Autodesk Inventor part; units mm, degrees
ref_plane "Work Plane1" through (6.76, 0, 0) normal (1, 0, 0) x (0, 1, 0)
ref_plane "XZ Plane" through (0, 0, 0) normal (0, 1, 0) x (-1, 0, 0)
ref_plane "XY Plane" through (0, 0, 0) normal (0, 0, 1) x (1, 0, 0)
sketch "Sketch1" plane through (0, 0, 0) normal (0, 1, 0) x (-1, 0, 0)
  circle A0 centre (0, 0) radius 11.5
  dimension "d0" = 23
extrude "Extrusion1" add sketch "Sketch1" along normal blind 1.5
sketch "Sketch2" plane through (0, 1.5, 0) normal (0, 1, 0) x (1, 0, 0)
  circle A0 centre (0, 0) radius 12.5
  dimension "d3" = 25
extrude "Extrusion2" add sketch "Sketch2" along normal blind 1.5
sketch "Sketch3" plane through (0, 0, 0) normal (0, -1, 0) x (1, 0, 0)
  circle A0 centre (0, 0) radius 12.5
  dimension "d6" = 25
extrude "Extrusion3" add sketch "Sketch3" along normal blind 1.5
sketch "Sketch4" plane through (0, -1.5, 0) normal (0, -1, 0) x (1, 0, 0)
  circle A0 centre (0, 0) radius 12.5
  line L0 (0, -12.5) -> (0, -9.5) construction
  circle A1 centre (0, -2.6096) radius 6.75
  circle A2 centre (0, -2.6096) radius 4
  dimension "d9" = 3
  dimension "d17" = 13.5
  dimension "d18" = 8
extrude "Extrusion6" add sketch "Sketch4" along normal blind 4.45 contours A1
extrude "Extrusion7" cut sketch "Sketch4" against normal blind 10 contours A2
ref_plane "Work Plane1" through (6.76, 0, 0) normal (1, 0, 0) x (0, 1, 0)
sketch "Sketch6" plane through (6.76, 0, 0) normal (1, 0, 0) x (0, 1, 0)
  line L0 (-5.95, 4.1404) -> (-5.95, -9.3596)
  line L1 (-1.5, -9.3596) -> (-1.5, 4.1404)
  line L2 (-5.95, -9.3596) -> (-5.95, 4.1404) construction
  line L3 (-1.5, -9.3596) -> (-5.95, -9.3596) construction
  line L4 (-5.95, 4.1404) -> (-1.5, 4.1404) construction
  line L5 (-1.5, 4.1404) -> (-5.95, 4.1404) construction
  line L6 (-5.95, -9.3596) -> (-5.95, -2.6096) construction
  line L7 (-5.95, 4.1404) -> (-3.725, 4.1404) construction
  line L8 (-3.725, 3.1248) -> (-3.725, -6.8752) construction
  circle A0 centre (-3.725, -2.6096) radius 0.8
  point P0 (0, 0)
  dimension "d24" = 4.45
  dimension "d25" = 13.5
  dimension "d26" = 6.75
  dimension "d27" = 2.225
  dimension "d28" = 10
  dimension "d29" = 1.6
extrude "Extrusion8" cut sketch "Sketch6" against normal blind 4.45
sketch "Sketch7" plane through (0, 3, 0) normal (0, 1, 0) x (1, 0, 0)
  circle A0 centre (0, 0) radius 11
  circle A1 centre (0, 2.6096) radius 4
  circle A2 centre (0, 2.6096) radius 4
  dimension "d32" = 22
extrude "Extrusion10" add sketch "Sketch7" along normal blind 0.2
properties part number "reverse gear eccentric 1"
Can you work these out from the model? Positions are in its coordinate system, mm. A direction names the side the tool comes from. Give positions to 0.01 mm unless a question says otherwise; leave off trailing zeros. Write each loop counter-clockwise with the first axis right and the second up, starting at its lowest first coordinate (ties: lowest second). Pieces come first, ordered by that corner, then holes. Notation, with made-up numbers: (-34.5, 72.25) -> (-15.5, 72.25) arc R22 cw to (-15.5, 93.25) -> close; hole circle Ø7 at (24, 60.5). An arc over 180 degrees is marked (long way). Answer as a JSON object with one key per item and string values. Group by question number.
Item 1: We'd pull the mould along Y, two halves only. Please class faces 4 (the face through (1.5, 0.7, -11.4)), 5 (the face through (11, 1.5, 4)), 6 (the face through (5, 3, 10)), 7 (the face through (3, -5.95, -6)): +Y half, -Y half, draft (parallel to the pull), parting line (faces both ways), or undercut.
Item 2: Suppose I cut it at D-D (z = 10.5). Please give me the cut outline in (x, y).
Item 3: I'm going to push flat-ended pins straight in: P1, Ø5, axis at x = 8.5, y = 0.5, coming from the -Z side; P2, Ø5, axis at y = -1, z = -8, coming from the +X side (3 decimals); P3, Ø4, axis at x = 5.5, y = -2.5, coming from the -Z side; P4, Ø6.5, axis at x = 0, z = -2.61, coming from the -Y side. Where does each tip first touch, or does it pass through?
Item 4: Suppose I cut it at C-C (x = 5.25). Please give me the cut outline in (y, z) (3 decimals).
Item 5: For faces 1 (the face through (3.63, -3.69, -8.3)), 2 (the face through (11, 0, -4)), 3 (the face through (5.35, -2.96, -2.37)), which set-ups out of +Z, -Z, +X, -X, +Y, -Y let a thin tool reach every point of the face, with its end or its side?
Item 6: Suppose I cut it at B-B (z = 0). Please give me the cut outline in (x, y).
Item 7: Please list where these lines run through material, in increasing order: line 1 (Z direction, x = 0, y = -2.75); line 2 (Z direction, x = 0, y = 0.75); line 3 (Y direction, x = 8, z = -8.5). Write a range as [from, to].
Item 8: Suppose I cut it at A-A (x = 0). Please give me the cut outline in (y, z).
Findings:
{
 "1": {"face 4": "undercut", "face 5": "undercut", "face 6": "+Y half", "face 7": "-Y half"},
 "2": {"outline": "(-6.78, -1.5) -> (6.78, -1.5) -> (6.78, 0) -> (4.69, 0) -> (4.69, 1.5) -> (6.78, 1.5) -> (6.78, 3) -> (3.28, 3) -> (3.28, 3.2) -> (-3.28, 3.2) -> (-3.28, 3) -> (-6.78, 3) -> (-6.78, 1.5) -> (-4.69, 1.5) -> (-4.69, 0) -> (-6.78, 0) -> close"},
 "3": {"P1": "stops at z = -10.94", "P2": "stops at x = 11.225", "P3": "stops at z = -11.92", "P4": "passes through"},
 "4": {"outline": "(-5.95, -6.852) -> (-1.5, -6.852) -> (-1.5, -11.344) -> (0, -11.344) -> (0, -10.232) -> (1.5, -10.232) -> (1.5, -11.344) -> (3, -11.344) -> (3, -9.666) -> (3.2, -9.666) -> (3.2, 9.666) -> (3, 9.666) -> (3, 11.344) -> (1.5, 11.344) -> (1.5, 10.232) -> (0, 10.232) -> (0, 11.344) -> (-1.5, 11.344) -> (-1.5, 1.633) -> (-5.95, 1.633) -> close; hole circle Ø1.6 at (-3.725, -2.61)"},
 "5": {"face 1": "-Y", "face 2": "none", "face 3": "+X"},
 "6": {"outline": "(-12.5, -1.5) -> (-6.23, -1.5) -> (-6.23, -5.95) -> (-3.03, -5.95) -> (-3.03, 3.2) -> (-11, 3.2) -> (-11, 3) -> (-12.5, 3) -> (-12.5, 1.5) -> (-11.5, 1.5) -> (-11.5, 0) -> (-12.5, 0) -> close; (3.03, -5.95) -> (6.23, -5.95) -> (6.23, -1.5) -> (12.5, -1.5) -> (12.5, 0) -> (11.5, 0) -> (11.5, 1.5) -> (12.5, 1.5) -> (12.5, 3) -> (11, 3) -> (11, 3.2) -> (3.03, 3.2) -> close"},
 "7": {"line 1": "z = [-9.36, -6.61], [1.39, 4.14]", "line 2": "z = [-11.5, -6.61], [1.39, 11.5]", "line 3": "y = [-1.5, 0], [1.5, 3]"},
 "8": {"outline": "(-5.95, -9.36) -> (-1.5, -9.36) -> (-1.5, -12.5) -> (0, -12.5) -> (0, -11.5) -> (1.5, -11.5) -> (1.5, -12.5) -> (3, -12.5) -> (3, -11) -> (3.2, -11) -> (3.2, -6.61) -> (-5.95, -6.61) -> close; (-5.95, 1.39) -> (3.2, 1.39) -> (3.2, 11) -> (3, 11) -> (3, 12.5) -> (1.5, 12.5) -> (1.5, 11.5) -> (0, 11.5) -> (0, 12.5) -> (-1.5, 12.5) -> (-1.5, 4.14) -> (-5.95, 4.14) -> close"}
}
